Autodesk Inventor part; units mm, degrees
ref_plane "YZ Plane" through (0, 0, 0) normal (1, 0, 0) x (0, 1, 0)
ref_plane "XZ Plane" through (0, 0, 0) normal (0, 1, 0) x (-1, 0, 0)
ref_plane "XY Plane" through (0, 0, 0) normal (0, 0, 1) x (1, 0, 0)
sketch "Sketch1" plane through (0, 0, 0) normal (0, 0, 1) x (1, 0, 0)
  line L0 (12.7, -25.4) -> (-12.7, -25.4)
  line L1 (-12.7, -25.4) -> (-12.7, 25.4)
  line L2 (-12.7, 25.4) -> (12.7, 25.4)
  line L3 (12.7, 25.4) -> (12.7, -25.4)
  line L4 (12.7, -25.4) -> (-12.7, 25.4) construction
  line L5 (-12.7, -25.4) -> (12.7, 25.4) construction
  line L6 (11.1125, -23.8125) -> (-11.1125, -23.8125)
  line L7 (-11.1125, -23.8125) -> (-11.1125, 23.8125)
  line L8 (-11.1125, 23.8125) -> (11.1125, 23.8125)
  line L9 (11.1125, 23.8125) -> (11.1125, -23.8125)
  line L10 (11.1125, -23.8125) -> (-11.1125, 23.8125) construction
  line L11 (-11.1125, -23.8125) -> (11.1125, 23.8125) construction
  point P0 (0, 0)
  dimension "d0" = 1.5875
  dimension "d1" = 1.5875
  dimension "d2" = 25.4
  dimension "d3" = 50.8
extrude "Extrusion1" add sketch "Sketch1" along normal mid plane 622.3
sketch "Sketch2" plane through (12.7, -25.4, 311.15) normal (1, 0, 0) x (0, 0, -1)
  line L0 (0, 0) -> (0, 50.8)
  line L1 (0, 50.8) -> (622.3, 50.8)
  point P0 (311.15, 25.4)
  point P1 (5, 25.4)
  point P2 (30.4, 25.4)
  point P3 (0, 25.4)
  point P4 (30.4, 13.97)
  point P5 (30.4, 39.37)
  dimension "d6" = 25.4
  dimension "d7" = 5
  dimension "d30" = 11.43
  dimension "d31" = 25.4
hole "Hole1" at (12.7, 0, 306.15) at (12.7, 0, 280.75) at (12.7, 13.97, 280.75) at (12.7, -11.43, 280.75) direction (-1, 0, 0) diameter 5.105 end through all
mirror "Mirror1" about plane through (0, 0, 0) normal (0, 0, 1) of "Hole1"
sketch "Sketch3" plane through (12.7, -25.4, 311.15) normal (1, 0, 0) x (0, 0, -1)
  line L0 (622.3, 0) -> (0, 0)
  point P0 (311.15, 25.4)
  point P1 (311.15, 25.4)
  point P2 (260.35, 25.4)
  point P3 (209.55, 25.4)
  point P4 (158.75, 25.4)
  point P5 (107.95, 25.4)
  point P6 (57.15, 25.4)
  point P7 (361.95, 25.4)
  point P8 (311.15, 25.4)
  point P9 (260.35, 25.4)
  point P10 (209.55, 25.4)
  point P11 (158.75, 25.4)
  point P12 (107.95, 25.4)
  point P13 (412.75, 25.4)
  point P14 (361.95, 25.4)
  point P15 (311.15, 25.4)
  point P16 (260.35, 25.4)
  point P17 (209.55, 25.4)
  point P18 (158.75, 25.4)
  point P19 (463.55, 25.4)
  point P20 (412.75, 25.4)
  point P21 (361.95, 25.4)
  point P22 (311.15, 25.4)
  point P23 (260.35, 25.4)
  point P24 (209.55, 25.4)
  point P25 (514.35, 25.4)
  point P26 (463.55, 25.4)
  point P27 (412.75, 25.4)
  point P28 (361.95, 25.4)
  point P29 (311.15, 25.4)
  point P30 (260.35, 25.4)
  point P31 (565.15, 25.4)
  point P32 (514.35, 25.4)
  point P33 (463.55, 25.4)
  point P34 (412.75, 25.4)
  point P35 (361.95, 25.4)
  point P36 (311.15, 25.4)
  dimension "d17" = 50.8
  dimension "d20" = 50.8
hole "Hole2" at (12.7, 0, 0) at (12.7, 0, 50.8) at (12.7, 0, 101.6) at (12.7, 0, 152.4) at (12.7, 0, 203.2) at (12.7, 0, 254) at (12.7, 0, -50.8) at (12.7, 0, -101.6) at (12.7, 0, -152.4) at (12.7, 0, -203.2) at (12.7, 0, -254) direction (-1, 0, 0) diameter 5.105 end through all
equation "\"d1\" = d0"
properties part number "CRASH_BAR_INTAKE" material "Aluminum, 6061-T6"
Verification items for the finished model (mm, model axes). A direction names the side the tool comes from. Round coordinates to 2 decimals unless told otherwise and drop trailing zeros. Loops run counter-clockwise (first coordinate to the right, second up) from the corner with the lowest first, then second, coordinate; pieces in that order, holes last. Notation, with made-up numbers: (-17.5, 35) -> (-1.5, 35) arc R18 ccw to (-1.5, 40) -> close; hole circle Ø9 at (85.5, 17). An arc over 180 degrees is marked (long way). Answer as a JSON object with one key per item and string values.
Q1. Scan lines: line 1 (Y direction, x = -12.15, z = 280.75); line 2 (X direction, y = -6, z = -211.5); line 3 (Y direction, x = -10.5, z = 133). Record each from-to range of solid material in increasing order. Write a range as from..to.
Data:
{"line 1": "y = -25.4..-13.98, -8.88..-2.55, 2.55..11.42, 16.52..25.4", "line 2": "x = -12.7..-11.11, 11.11..12.7", "line 3": "y = -25.4..-23.81, 23.81..25.4"}
Q2. Section check B-B (x = -6.75). Record the boundary of the cut face in (y, z).
Data:
{"outline": "(-25.4, -311.15) -> (-23.81, -311.15) -> (-23.81, 311.15) -> (-25.4, 311.15) -> close; (23.81, -311.15) -> (25.4, -311.15) -> (25.4, 311.15) -> (23.81, 311.15) -> close"}
Q3. Section check A-A (z = 8). Record the boundary of the cut face in (x, y), then the cut area to 3 significant figures.
Data:
{"outline": "(-12.7, -25.4) -> (12.7, -25.4) -> (12.7, 25.4) -> (-12.7, 25.4) -> close; hole (-11.11, -23.81) -> (11.11, -23.81) -> (11.11, 23.81) -> (-11.11, 23.81) -> close", "area": "232 mm2"}
Q4. Draft check along Y on faces 1 (the flat face through (-11.3, 2, -311.15)), 2 (the flat face through (0, -25.4, -4)), 3 (the flat face through (0, -23.812, -4)). Enter one of: pulls with the +Y half, pulls with the -Y half, needs draft (parallel to the pull), parting line crosses it, or undercut.
Data:
{"face 1": "needs draft", "face 2": "pulls with the -Y half", "face 3": "undercut"}
Q5. Access from +Z, -Z, +X, -X, +Y, -Y to the whole of each face (thin tool, end or side, straight path). Record for faces 4 (the flat face through (11.112, 0, -4)), 5 (the flat face through (12.7, 0, -4)).
Data:
{"face 4": "+Z, -Z", "face 5": "+Z, -Z, +X, +Y, -Y"}
